Design review of the part built by this model. Coordinates are the model's own, in mm. A direction names the side the tool comes from. Coordinates: 2 decimals unless noted, no trailing zeros. Write each loop counter-clockwise with the first axis right and the second up, starting at its lowest first coordinate (ties: lowest second). Pieces come first, ordered by that corner, then holes. Notation, with made-up numbers: (-2.75, 67) - (39.25, 67) arc R6 ccw to (39.25, 75) - close; hole circle Ø2 at (5.5, 39.25). An arc over 180 degrees is marked (long way). Use a Markdown table: item, result.
from build123d import *

# Parameters (mm, degrees)
SKETCH1_R           = 34
BOSS_EXTRUDE1_DEPTH = 6
CIRPATTERN1_COUNT   = 4
SKETCH5_R           = 12.5
CUT_EXTRUDE1_DEPTH  = 49.456165758
SKETCH7_W           = 18
SKETCH7_H           = 56.5
CUT_EXTRUDE4_DEPTH  = 49.456165758


with BuildPart() as part:
    # Sketch1 → Boss-Extrude1 (new body)
    with BuildSketch(Plane(origin=(0, 0, 0), x_dir=(1, 0, 0), z_dir=(0, 1, 0))):
        with Locations(Location((0, 0, 0), (0, 0, 270))):
            Circle(SKETCH1_R)
    extrude(amount=BOSS_EXTRUDE1_DEPTH)

    # Sketch3 → Hole1 (revolve, cut)
    with BuildSketch(Plane(origin=(17.324, 6, -17.324), x_dir=(0, 0, 1), z_dir=(1, 0, 0))):
        Polygon((0, 0), (0, 11.502151548), (2.5, 10), (2.5, 0), align=None)
    hole1 = revolve(axis=Axis((17.324, 12.35, -17.324), (0, -1, 0)), mode=Mode.SUBTRACT)

    # CirPattern1: Hole1 ×4 about axis
    cirpattern1_axis = Axis((0, 0, 0), (0, 1, 0))
    for i in range(1, CIRPATTERN1_COUNT):
        add(hole1.rotate(cirpattern1_axis, i * 360 / CIRPATTERN1_COUNT), mode=Mode.SUBTRACT)

    # Sketch5 → Cut-Extrude1 (cut, through all)
    with BuildSketch(Plane(origin=(0, 6, 0), x_dir=(1, 0, 0), z_dir=(0, 1, 0))):
        with Locations(Location((0, 0, 0), (0, 0, 270))):
            Circle(SKETCH5_R)
    extrude(amount=-CUT_EXTRUDE1_DEPTH, mode=Mode.SUBTRACT)

    # Sketch7 → Cut-Extrude4 (cut, through all)
    with BuildSketch(Plane(origin=(0, 0, 0), x_dir=(1, 0, 0), z_dir=(0, 1, 0))):
        with Locations((0, -51.75)):
            Rectangle(SKETCH7_W, SKETCH7_H)
    extrude(amount=CUT_EXTRUDE4_DEPTH, mode=Mode.SUBTRACT)


solid = part.part
(1) Take a section at B-B on z = 0. Write out the cut boundary in (x, y), and give its area (3 significant figures).
Determined:
| item | result |
|---|---|
| outline | (-34, 0) - (-12.5, 0) - (-12.5, 6) - (-34, 6) - close; (12.5, 0) - (34, 0) - (34, 6) - (12.5, 6) - close |
| area | 258 mm2 |
(2) Machinability: for faces 1 (the flat face through (9, 3, 28)), 2 (the cylindrical face through (-19.167, 3.042, -15.634)), which of the approach directions +Z, -Z, +X, -X, +Y, -Y give a long, thin tool a straight path to every point of the face, cutting with its end or side? Answer none if there is none.
Determined:
| item | result |
|---|---|
| face 1 | +Z, +Y, -Y |
| face 2 | +Y, -Y |
(3) Take a section at A-A on x = 0. Write out the cut boundary in (y, z).
Determined:
| item | result |
|---|---|
| outline | (0, -34) - (6, -34) - (6, -12.5) - (0, -12.5) - close; (0, 12.5) - (6, 12.5) - (6, 23.5) - (0, 23.5) - close |
(4) Take a section at D-D on x = -18.5. Write out the cut boundary in (y, z), and give its area (3 significant figures).
Determined:
| item | result |
|---|---|
| outline | (0, -28.53) - (6, -28.53) - (6, -19.53) - (0, -19.53) - close; (0, -15.12) - (6, -15.12) - (6, 15.12) - (0, 15.12) - close; (0, 19.53) - (6, 19.53) - (6, 28.53) - (0, 28.53) - close |
| area | 289 mm2 |
(5) For L1, parallel to X at y = 4.15, z = -19; L2, parallel to X at y = 3.3, z = 0; L3, parallel to X at y = 3.25, z = 19.5, list the stretches that pass through material, from the lowest coordinate up. Write a range as from..to.
Determined:
| item | result |
|---|---|
| L1 | -28.2..-19.18, -15.47..15.47, 19.18..28.2 |
| L2 | -34..-12.5, 12.5..34 |
| L3 | -27.85..-18.55, -16.09..16.09, 18.55..27.85 |
(6) Draft analysis for pull direction Z (two halves, no side actions). For faces 3 (the cylindrical face through (-15.634, 3.042, 19.167)), 4 (the flat face through (-15, 0, -1)), 5 (the flat face through (0, 3, 23.5)), state which applies: +Z half, -Z half, draft (parallel to the pull), parting line (faces both ways), or undercut.
Determined:
| item | result |
|---|---|
| face 3 | undercut |
| face 4 | draft |
| face 5 | +Z half |
(7) For pin 1 (1 mm diameter, centred on x = -8.5, y = 2, fed in from -Z); pin 2 (1.8 mm diameter, centred on y = 2.5, z = 30, fed in from -X); pin 3 (1.8 mm diameter, centred on y = 3.5, z = 30.5, fed in from +X), all flat-tipped, find the tip position at first contact; note any pin that passes through.
Determined:
| item | result |
|---|---|
| pin 1 | z = -33.05 |
| pin 2 | x = -17.58 |
| pin 3 | x = 16.73 |
(8) Take a section at C-C on z = 18.5. Write out the cut boundary in (x, y).
Determined:
| item | result |
|---|---|
| outline | (-28.53, 0) - (-19.53, 0) - (-19.53, 6) - (-28.53, 6) - close; (-15.12, 0) - (15.12, 0) - (15.12, 6) - (-15.12, 6) - close; (19.53, 0) - (28.53, 0) - (28.53, 6) - (19.53, 6) - close |
